Build history of the part. All positions in model axes, mm. A direction names the side the tool comes from. Round coordinates to 2 decimals unless told otherwise and drop trailing zeros. Order: outer loops, then holes, each group sorted by start corner. A loop starts at its lowest first (then second) coordinate and runs counter-clockwise, first axis right, second up. Notation, with made-up numbers: (6, -24) -> (56, -24) arc R29 ccw to (56, -4) -> close; hole circle Ø11 at (86.5, -4.5). An arc over 180 degrees is marked (long way). Use a Markdown table: item, result. Add a question column.
Item 1: Slice it at B-B, the plane y = 2.25. Give the cut face in (x, z).
Item 2: Probe L1, parallel to X at y = 10.75, z = 1.75; L2, parallel to X at y = 2.75, z = 0.55; L3, parallel to X at y = 3.5, z = 2.5. List the from-to ranges inside material, lowest first.
Item 3: Slice it at C-C, the plane y = 12.5. Give the cut face in (x, z), plus the area to 3 significant figures.
Item 4: Slice it at A-A, the plane y = 6.5. Give the cut face in (x, z), plus the area to 3 significant figures.
Item 5: Slice it at D-D, the plane x = -18.25. Give the cut face in (y, z).
Item 6: 3-axis set-ups, long thin cutter, end or side, ignore diameter. For faces 1 (the face through (0, 2, 2)), 2 (the face through (-20, 2, 1)), 3 (the face through (-16.5, 4, 1)), 4 (the face through (-19, 13, 1)): which of +Z, -Z, +X, -X, +Y, -Y reach the whole face in a straight line?
Item 7: Two-plate mould, pull along X, no slides. Class faces 5 (the face through (0, 10, 2)), 6 (the face through (-4, 4, 1)), 7 (the face through (-8, 14.693, 2)): released by +X, released by -X, zero draft, split by the parting line, or undercut.
Item 8: Pin check, flat tips, straight feed: pin 1 (0.9 mm diameter, centred on y = 11, z = 2, fed in from +X); pin 2 (1.6 mm diameter, centred on x = -19, z = 1.5, fed in from +Y); pin 3 (1.5 mm diameter, centred on y = 2.5, z = 1.5, fed in from +X). Stop position of each tip, or through.
Autodesk Inventor part; units mm, degrees
ref_plane "YZ Plane" through (0, 0, 0) normal (1, 0, 0) x (0, 1, 0)
ref_plane "XZ Plane" through (0, 0, 0) normal (0, 1, 0) x (-1, 0, 0)
ref_plane "XY Plane" through (0, 0, 0) normal (0, 0, 1) x (1, 0, 0)
sketch "Sketch1" plane through (0, 0, 0) normal (0, 1, 0) x (-1, 0, 0)
  line L0 (0, 0) -> (20, 0)
  line L1 (20, 0) -> (20, 3)
  line L2 (20, 3) -> (0, 3)
  line L3 (0, 3) -> (0, 0)
  dimension "d0" = 20
  dimension "d1" = 3
extrude "Extrusion1" add sketch "Sketch1" along normal blind 10
sketch "Sketch2" plane through (0, 10, 0) normal (0, 1, 0) x (1, 0, 0)
  line L0 (-20, 0) -> (-20, -3)
  line L1 (0, 0) -> (-20, 0)
  line L2 (-20, -3) -> (0, -3)
  line L3 (0, -3) -> (0, 0)
  line L4 (-14.5, 0) -> (-10.5, 0)
  line L5 (-10.5, 0) -> (-10.5, -3)
  line L6 (-10.5, -3) -> (-14.5, -3)
  line L7 (-14.5, -3) -> (-14.5, 0)
  line L8 (-9.5, 0) -> (-5.5, 0)
  line L9 (-5.5, 0) -> (-5.5, -3)
  line L10 (-5.5, -3) -> (-9.5, -3)
  line L11 (-9.5, -3) -> (-9.5, 0)
  line L12 (-10, 1.8071) -> (-10, -4.5751) construction
  dimension "d26" = 20
  dimension "d27" = 4
  dimension "d28" = 4
  dimension "d45" = 1
  dimension "d46" = 10
  dimension "d47" = 0.5
extrude "Extrusion2" add sketch "Sketch2" along normal blind 3 contours L1 L5 L2 L7 | L1 L9 L2 L11
sketch "Sketch5" plane through (0, 0, 0) normal (0, 0, -1) x (-1, 0, 0)
  line L0 (0, 0) -> (20, 0)
  line L1 (9.5, 10) -> (10.5, 10)
  line L2 (16.2, 7.5) -> (16.3, 7.5)
  line L3 (16.5, 7.3) -> (16.5, 0)
  line L4 (16.5, 0) -> (16, 0)
  line L5 (16, 0) -> (16, 7.3)
  line L6 (10, 10) -> (10, 0) construction
  arc A0 (16.2, 7.5) -> (16, 7.3) centre (16.2, 7.3) ccw
  arc A1 (16.5, 7.3) -> (16.3, 7.5) centre (16.3, 7.3) ccw
  line L7 (3.8, 7.5) -> (3.7, 7.5)
  line L8 (3.5, 7.3) -> (3.5, 0)
  line L9 (3.5, 0) -> (4, 0)
  line L10 (4, 0) -> (4, 7.3)
  arc A2 (4, 7.3) -> (3.8, 7.5) centre (3.8, 7.3) ccw
  arc A3 (3.7, 7.5) -> (3.5, 7.3) centre (3.7, 7.3) ccw
  point P0 (16.5, 7.5)
  point P1 (3.5, 7.5)
  dimension "d61" = 0.5
  dimension "d62" = 7.5
  dimension "d63" = 6
  dimension "d64" = 0.2
extrude "Extrusion5" cut sketch "Sketch5" against normal blind 3
sketch "Sketch6" plane through (-20, 0, 0) normal (0, 0, -1) x (-1, 0, 0)
  line L0 (0, 0) -> (0, 10)
  line L1 (-5.5, 10) -> (0, 10)
  line L2 (-10.5, 10) -> (-9.5, 10)
  line L3 (-2.75, 10) -> (-2.75, 5) construction
  line L4 (-2.75, 5) -> (0, 5) construction
  line L5 (0, 5) -> (0.7, 5)
  line L6 (0, 5) -> (0, 7)
  line L7 (0, 7) -> (0.5844, 5.3304)
  line L8 (0, 5) -> (0, 3)
  line L9 (0, 3) -> (0.5844, 4.6696)
  arc A0 (0.5844, 4.6696) -> (0.5844, 5.3304) centre (-0.3595, 5) ccw
  line L10 (-16.5, 0) -> (-16.5, 7.3)
  line L11 (-16, 7.3) -> (-16, 0)
  line L12 (-10, 10) -> (-10, 0) construction
  line L13 (-20, 5) -> (-20, 7)
  line L14 (-20, 7) -> (-20.5844, 5.3304)
  line L15 (-20, 5) -> (-20, 3)
  line L16 (-20, 3) -> (-20.5844, 4.6696)
  arc A1 (-20.5844, 5.3304) -> (-20.5844, 4.6696) centre (-19.6405, 5) ccw
  dimension "d36" = 5
  dimension "d37" = 0.7
  dimension "d38" = 2
  dimension "d39" = 2
  dimension "d40" = 1
extrude "Extrusion6" add sketch "Sketch6" against normal blind 3
sketch "Sketch7" plane through (-5.5, 10, 3) normal (0, 0, 1) x (1, 0, 0)
  line L0 (-5, 0) -> (-4, 0)
  line L1 (-9, 3) -> (-5, 3)
  line L2 (-9, 0) -> (-9, 3)
  line L3 (-14.5, -10) -> (-11, -10)
  line L4 (-9, 3) -> (-9.5, 3)
  line L5 (-9.5, 3) -> (-9, 4.6927)
  line L6 (-9, 4.6927) -> (-5, 4.6927)
  line L7 (-5, 4.6927) -> (-5, 3)
  line L8 (-4.5, 0) -> (-4.5, 8.186) construction
  line L9 (0, 3) -> (-4, 3)
  line L10 (0, 3) -> (0.5, 3)
  line L11 (0.5, 3) -> (0, 4.6927)
  line L12 (0, 4.6927) -> (-4, 4.6927)
  line L13 (-4, 4.6927) -> (-4, 3)
  line L14 (-4.5, 0) -> (-4.5, -4) construction
  line L15 (-5, 0) -> (-4.5, -4)
  line L16 (-4, 0) -> (-4.5, -4)
  point P0 (-9, -10)
  dimension "d48" = 0.5
  dimension "d49" = 4
extrude "Extrusion7" add sketch "Sketch7" against normal blind 3 contours L4 L5 L6 L7 L1 | L9 L13 L12 L11 L10
extrude "Extrusion8" cut sketch "Sketch7" against normal blind 3 contours L0 L16 L15
fillet "Fillet1" radius 1 2 edges at (-5.5, 14.6927, 1.5) (-14.5, 14.6927, 1.5)
sketch "Sketch8" plane through (0, 10, 0) normal (0, 1, 0) x (1, 0, 0)
  line L0 (0, -3) -> (0, 0)
  line L1 (0, 0) -> (-5.5, 0)
  line L2 (-14.5, -3) -> (-14.5, 0)
  line L3 (-14.5, 0) -> (-20, 0)
  line L4 (-20, 0) -> (-20, -3)
  line L5 (-20, -3) -> (-14.5, -3)
  line L6 (-20, 0) -> (-18, 0)
  line L7 (-18, 0) -> (-18, -3)
  line L8 (-18, -3) -> (-20, -3)
  line L9 (-20, -3) -> (-20, 0)
  line L10 (-20, 0) -> (-20, -3)
  line L11 (-14.5, 0) -> (-20, 0)
  line L12 (-2, 0) -> (0, 0)
  line L13 (0, 0) -> (0, -3)
  line L14 (0, -3) -> (-2, -3)
  line L15 (-2, -3) -> (-2, 0)
  dimension "d55" = 2
  dimension "d56" = 3
  dimension "d57" = 2
  dimension "d58" = 3
extrude "Extrusion9" add sketch "Sketch8" along normal blind 3 contours L14 L15 L1 L0 | L5 L4 L3 L7
fillet "Fillet2" radius 1 2 edges at (0, 0, 1.5) (-20, 0, 1.5)
equation "\"d28\" = d27"
equation "\"d46\" = 0.5 * d26"
equation "\"d47\" = 0.5 * d45"
equation "\"d39\" = d38"
properties part number "pressfit1press" material "Glass"
Check sheet entries:
| question | item | result |
|---|---|---|
| 1 | outline | (-20, 0) -> (-16.5, 0) -> (-16.5, 3) -> (-20, 3) -> close; (-16, 0) -> (-4, 0) -> (-4, 3) -> (-16, 3) -> close; (-3.5, 0) -> (0, 0) -> (0, 3) -> (-3.5, 3) -> close |
| 2 | L1 | -20 to -18, -14.5 to -10.5, -9.5 to -5.5, -2 to 0 |
| 2 | L2 | -20 to -16.5, -16 to -4, -3.5 to 0 |
| 2 | L3 | -20.18 to -16.5, -16 to -4, -3.5 to 0.18 |
| 3 | outline | (-20, 0) -> (-18, 0) -> (-18, 3) -> (-20, 3) -> close; (-14.5, 0) -> (-10.5, 0) -> (-10.5, 3) -> (-14.5, 3) -> close; (-9.5, 0) -> (-5.5, 0) -> (-5.5, 3) -> (-9.5, 3) -> close; (-2, 0) -> (0, 0) -> (0, 3) -> (-2, 3) -> close |
| 3 | area | 36.0 mm2 |
| 4 | outline | (-20.18, 0) -> (-16.5, 0) -> (-16.5, 3) -> (-20.18, 3) -> close; (-16, 0) -> (-10.06, 0) -> (-10.06, 3) -> (-16, 3) -> close; (-9.94, 0) -> (-4, 0) -> (-4, 3) -> (-9.94, 3) -> close; (-3.5, 0) -> (0.18, 0) -> (0.18, 3) -> (-3.5, 3) -> close |
| 4 | area | 57.7 mm2 |
| 5 | outline | (0, 0) -> (13, 0) -> (13, 3) -> (0, 3) -> close |
| 6 | face 1 | +Z, -Z, +X, -Y |
| 6 | face 2 | +Z, -Z, -X, -Y |
| 6 | face 3 | +Z, -Z, -Y |
| 6 | face 4 | +Z, -Z, -X, +Y |
| 7 | face 5 | released by +X |
| 7 | face 6 | undercut |
| 7 | face 7 | zero draft |
| 8 | pin 1 | x = 0 |
| 8 | pin 2 | y = 13 |
| 8 | pin 3 | x = 0.09 |
